from build123d import *

# Parameters (mm, degrees)
SKETCH2_W          = 11.43
SKETCH2_H          = 11.43
CENTRAL_BOX_DEPTH  = 10.16
NIBBLES_DEPTH      = 6.35
NIBBLES_DEPTH_BACK = 16.51
SKETCH4_R          = 3.175
YAY_ROUNDED_R      = 2.54


with BuildPart() as part:
    # Sketch2 → central box (new body)
    with BuildSketch(Plane(origin=(0, 0, 0), x_dir=(0, 0, -1), z_dir=(1, 0, 0))):
        with Locations((5.715, 5.715)):
            Rectangle(SKETCH2_W, SKETCH2_H)
    extrude(amount=CENTRAL_BOX_DEPTH)

    # Sketch4 → nibbles (add, two sides: drawn at the far end of the back side and taken through both)
    with BuildSketch(Plane(origin=(10.16, 0, 0), x_dir=(0, 0, -1), z_dir=(1, 0, 0)).offset(-NIBBLES_DEPTH_BACK)):
        with Locations(Location((5.715, 5.715, 0), (0, 0, 180))):
            Circle(SKETCH4_R)
    extrude(amount=NIBBLES_DEPTH + NIBBLES_DEPTH_BACK)

    # Sketch6 → stick (revolve)
    with BuildSketch(Plane.XY.offset(-5.715), mode=Mode.PRIVATE) as stick_sk:
        with BuildLine():
            Line((5.08, 11.43), (5.08, 39.37))
            Line((5.08, 39.37), (17.007592302, 39.37))
            Line((17.007592302, 39.37), (17.007592302, 34.29))
            add(Edge.make_bspline(
                [(17.007592302, 34.29), (5.959076516, 41.944088777), (10.418992682, 27.645249109), (7.112, 11.43)],
                knots=[0, 0, 0, 0, 1, 1, 1, 1], degree=3))
            Line((7.112, 11.43), (5.08, 11.43))
        make_face()
    revolve(stick_sk.sketch.rotate(Axis((5.08, 11.43, -5.715), (0, 1, 0)), 90), axis=Axis((5.08, 11.43, -5.715), (0, 1, 0)))

    # yay, rounded
    yay_rounded_edges = [part.edges().sort_by_distance(p)[0] for p in [
        (0, 5.715, -8.89),
        (10.16, 5.715, -8.89),
        (5.08, 11.43, -3.683),
        (5.08, 39.37, 6.212592302),
    ]]
    fillet(yay_rounded_edges, radius=YAY_ROUNDED_R - 0.0001)  # a hair under: the kernel refuses the full size


solid = part.part
Here's how the part is built. I have some questions about the finished solid (model axes, mm). A direction names the side the tool comes from. Coordinates: 2 decimals unless noted, no trailing zeros.
1. For P1, Ø1, axis at x = 0, y = 9.5, coming from the -Z side; P2, Ø1.9, axis at y = 6, z = -5, coming from the -X side; P3, Ø12.5, axis at y = 7.5, z = -6, coming from the +X side, each with a flat end and sliding along its axis, tell me the tip position at first contact or that it passes through.
2. For faces 4 (the cylindrical face through (-4.472, 2.567, -6.128)), 5 (the flat face through (5, 6, 0)), 6 (the flat face through (-6.35, 6, -6)), which set-ups out of +Z, -Z, +X, -X, +Y, -Y let a thin tool reach every point of the face, with its end or its side?
3. I need wall thicknesses on L1, parallel to X at y = 35.5, z = -2.5; L2, parallel to Z at x = 12.5, y = 35; L3, parallel to Y at x = -5.25, z = -3.75. Which ranges of each line are inside material? Lowest first, please.
4. If we mould it in two halves opening along Y, with no side actions, what happens to faces 1 (the flat face through (0, 11, -3)), 2 (the flat face through (5, 39.37, -6)), 3 (the flat face through (16.51, 6, -6))? For each: pulls with the +Y half, pulls with the -Y half, needs draft (parallel to the pull), parting line crosses it, or undercut.
Taken from the geometry:
1. P1: stops at z = -11.43
1. P2: stops at x = -6.35
1. P3: stops at x = 16.51
2. face 4: -X
2. face 5: +Z, +X, -X, -Y
2. face 6: +Z, -Z, -X, -Y
3. L1: x = -6.41 to -4.37, 0.89 to 9.27, 14.53 to 16.57
3. L2: z = -15.05 to -13.63, 2.2 to 3.62
3. L3: y = 3.22 to 8.21, 35.2 to 39.11
4. face 1: undercut
4. face 2: pulls with the +Y half
4. face 3: needs draft
